The model under review builds one solid part; all positions refer to its coordinate system, in mm. A direction names the side the tool comes from. Give positions to 0.01 mm unless a question says otherwise; leave off trailing zeros. Order: outer loops, then holes, each group sorted by start corner. A loop starts at its lowest first (then second) coordinate and runs counter-clockwise, first axis right, second up. Notation, with made-up numbers: (18.5, 35.25) -> (55.5, 35.25) arc R20 ccw to (55.5, 50.25) -> close; hole circle Ø4 at (5, 54). An arc over 180 degrees is marked (long way). Answer as a JSON object with one key per item and string values. Group by question number.
from build123d import *

# Parameters (mm, degrees)
F0_W     = 168.91
F0_H     = 127
F1_DEPTH = 12.7
F2_W     = 6.35
F2_H     = 101.6
F3_DEPTH = 12.7
F4_R     = 45.84191
F5_DEPTH = 25.4


with BuildPart() as f1:
    # F0 (on Top) → F1 (new body)
    with BuildSketch(Plane.XY):
        Rectangle(F0_W, F0_H)
    extrude(amount=F1_DEPTH)

    # F2 (on face) → F3 (join)
    with BuildSketch(Plane.XY.offset(12.7)):
        with Locations((68.58, 0)):
            Rectangle(F2_W, F2_H)
        with Locations((-68.58, 0)):
            Rectangle(F2_W, F2_H)
    extrude(amount=F3_DEPTH)

    # F4 (on Top) → F5 (cut)
    with BuildSketch(Plane.XY):
        Circle(F4_R)
    extrude(amount=F5_DEPTH, mode=Mode.SUBTRACT)


solid = f1.part
1. For pin 1 (3 mm diameter, centred on x = 68, z = 18, fed in from -Y); pin 2 (10 mm diameter, centred on y = 6.5, z = 21.5, fed in from +X) (3 decimals); pin 3 (10 mm diameter, centred on y = -13.5, z = 20, fed in from -X) (3 decimals); pin 4 (12 mm diameter, centred on y = -19, z = 16, fed in from -X) (3 decimals), all flat-tipped, find the tip position at first contact; note any pin that passes through.
2. Draft analysis for pull direction X (two halves, no side actions). For faces 1 (the flat face through (65.405, -1, 19)), 2 (the flat face through (84.455, -1, 6)), 3 (the flat face through (-1, -63.5, 6)), state which applies: pulls with the +X half, pulls with the -X half, needs draft (parallel to the pull), parting line crosses it, or undercut.
3. Take a section at B-B on y = 0. Give the boundary of the cut face in (x, z) (3 decimals).
4. Machinability: for faces 4 (the flat face through (-71.755, -1, 19)), 5 (the flat face through (71.755, -1, 19)), 6 (the flat face through (-65.405, -1, 19)), 7 (the flat face through (-69, 50.8, 19)), which of the approach directions +Z, -Z, +X, -X, +Y, -Y give a long, thin tool a straight path to every point of the face, cutting with its end or side? Answer none if there is none.
5. Take a section at C-C on z = 19.75. Give the boundary of the cut face in (x, y) (3 decimals), plus the area to 3 significant figures.
6. Take a section at A-A on x = 0. Give the boundary of the cut face in (y, z), plus the area to 3 significant figures.
7. Take a section at D-D on z = 8. Give the boundary of the cut face in (x, y) (3 decimals).
8. For probe 1 along X at (y, z) = (-46, 16) (3 decimals); probe 2 along Y at (x, z) = (0, 8.75); probe 3 along X at (y, z) = (0, 8.5) (3 decimals), list the stretches that pass through material, from the lowest coordinate up. Write a range as [from, to].
Checks:
{
 "1": {"pin 1": "stops at y = -50.8", "pin 2": "stops at x = 71.755", "pin 3": "stops at x = -71.755", "pin 4": "stops at x = -84.455"},
 "2": {"face 1": "undercut", "face 2": "pulls with the +X half", "face 3": "needs draft"},
 "3": {"outline": "(-84.455, 0) -> (-45.842, 0) -> (-45.842, 12.7) -> (-65.405, 12.7) -> (-65.405, 25.4) -> (-71.755, 25.4) -> (-71.755, 12.7) -> (-84.455, 12.7) -> close; (45.842, 0) -> (84.455, 0) -> (84.455, 12.7) -> (71.755, 12.7) -> (71.755, 25.4) -> (65.405, 25.4) -> (65.405, 12.7) -> (45.842, 12.7) -> close"},
 "4": {"face 4": "+Z, -X, +Y, -Y", "face 5": "+Z, +X, +Y, -Y", "face 6": "+Z, +Y, -Y", "face 7": "+Z, +X, -X, +Y"},
 "5": {"outline": "(-71.755, -50.8) -> (-65.405, -50.8) -> (-65.405, 50.8) -> (-71.755, 50.8) -> close; (65.405, -50.8) -> (71.755, -50.8) -> (71.755, 50.8) -> (65.405, 50.8) -> close", "area": "1,290 mm2"},
 "6": {"outline": "(-63.5, 0) -> (-45.84, 0) -> (-45.84, 12.7) -> (-63.5, 12.7) -> close; (45.84, 0) -> (63.5, 0) -> (63.5, 12.7) -> (45.84, 12.7) -> close", "area": "449 mm2"},
 "7": {"outline": "(-84.455, -63.5) -> (84.455, -63.5) -> (84.455, 63.5) -> (-84.455, 63.5) -> close; hole circle Ø91.684 at (0, 0)"},
 "8": {"probe 1": "x = [-71.755, -65.405], [65.405, 71.755]", "probe 2": "y = [-63.5, -45.84], [45.84, 63.5]", "probe 3": "x = [-84.455, -45.842], [45.842, 84.455]"}
}
